For this review, take the finished solid that the model builds, in its own axes (mm). A direction names the side the tool comes from. Coordinates: 2 decimals unless noted, no trailing zeros. Order: outer loops, then holes, each group sorted by start corner. A loop starts at its lowest first (then second) coordinate and runs counter-clockwise, first axis right, second up. Notation, with made-up numbers: (73, -22.5) -> (103, -22.5) arc R5 cw to (103, -14.5) -> close; hole circle Ø11 at (75, 12). An arc over 180 degrees is marked (long way). Return JSON: item names as keys, results as strings. Group by question number.
Item 1: Take a section at B-B (y = 40). Write out the cut boundary in (x, z).
Item 2: Take a section at C-C (x = 40). Write out the cut boundary in (y, z), then the cut area to 3 significant figures.
Item 3: For line 1 along Y through (x, z) = (40, 5.5); line 2 along X through (y, z) = (40, 5.75); line 3 along Y through (x, z) = (72.5, 4.5), list the stretches that pass through material, from the lowest coordinate up.
Item 4: Machinability: for faces 4 (the flat face through (2, 33.5, 7)), 5 (the cylindrical face through (21.502, 64.787, 6.549)), 6 (the cylindrical face through (2, 79, 5)), which of the approach directions +Z, -Z, +X, -X, +Y, -Y give a long, thin tool a straight path to every point of the face, cutting with its end or side? Answer none if there is none.
Item 5: Take a section at A-A (z = 7.25). Write out the cut boundary in (x, y).
Item 6: Take a section at D-D (x = 73). Write out the cut boundary in (y, z).
Item 7: Draft analysis for pull direction Y (two halves, no side actions). For faces 1 (the flat face through (38, 41, 3)), 2 (the flat face through (40, 80, 5)), 3 (the flat face through (80, 40, 5)), state which applies: +Y half, -Y half, draft (parallel to the pull), parting line (faces both ways), or undercut.
Item 8: Insertion check: pin 1 (1.8 mm diameter, centred on x = 2, z = 6, fed in from -Y). The pin has a flat end and moves straight along its axis. Give the tip position at first contact, or say it passes through.
```python
from build123d import *

# Parameters (mm, degrees)
F1_DEPTH = 10
F3_DEPTH = 7
F4_R     = 37
F4_R_2   = 35.5
F5_DEPTH = 7
F6_W     = 20.75
F6_H     = 14
F7_DEPTH = 7


with BuildPart() as f1:
    # F0 (on Top) → F1 (new body)
    with BuildSketch(Plane.XY):
        with BuildLine():
            Line((75, 80), (5, 80))
            ThreePointArc((5, 80), (1.464466, 78.535534), (0, 75))
            Line((0, 75), (0, 5))
            ThreePointArc((0, 5), (1.464466, 1.464466), (5, 0))
            Line((5, 0), (75, 0))
            ThreePointArc((75, 0), (78.535534, 1.464466), (80, 5))
            Line((80, 5), (80, 75))
            ThreePointArc((80, 75), (78.535534, 78.535534), (75, 80))
        make_face()
    extrude(amount=F1_DEPTH)

    # F2 (on face) → F3 (cut)
    with BuildSketch(Plane.XY.offset(10)):
        with BuildLine():
            ThreePointArc((20.75, 17), (21.482233, 15.232233), (23.25, 14.5))
            Line((23.25, 14.5), (57.75, 14.5))
            ThreePointArc((57.75, 14.5), (59.517767, 15.232233), (60.25, 17))
            Line((60.25, 17), (60.25, 63))
            ThreePointArc((60.25, 63), (59.517767, 64.767767), (57.75, 65.5))
            Line((57.75, 65.5), (23.25, 65.5))
            ThreePointArc((23.25, 65.5), (21.482233, 64.767767), (20.75, 63))
            Line((20.75, 63), (20.75, 17))
        make_face()
    extrude(amount=-F3_DEPTH, mode=Mode.SUBTRACT)

    # F4 (on face) → F5 (cut)
    with BuildSketch(Plane.XY.offset(10)):
        with Locations((40, 40)):
            Circle(F4_R)
        with Locations((40, 40)):
            Circle(F4_R_2, mode=Mode.SUBTRACT)
    extrude(amount=-F5_DEPTH, mode=Mode.SUBTRACT)

    # F6 (on face) → F7 (cut)
    with BuildSketch(Plane.XY.offset(10)):
        with Locations((10.375, 26.5)):
            Rectangle(F6_W, F6_H)
    extrude(amount=-F7_DEPTH, mode=Mode.SUBTRACT)


solid = f1.part
```
Findings below:
{
 "1": {"outline": "(0, 0) -> (80, 0) -> (80, 10) -> (77, 10) -> (77, 3) -> (75.5, 3) -> (75.5, 10) -> (60.25, 10) -> (60.25, 3) -> (20.75, 3) -> (20.75, 10) -> (4.5, 10) -> (4.5, 3) -> (3, 3) -> (3, 10) -> (0, 10) -> close"},
 "2": {"outline": "(0, 0) -> (80, 0) -> (80, 10) -> (77, 10) -> (77, 3) -> (75.5, 3) -> (75.5, 10) -> (65.5, 10) -> (65.5, 3) -> (14.5, 3) -> (14.5, 10) -> (4.5, 10) -> (4.5, 3) -> (3, 3) -> (3, 10) -> (0, 10) -> close", "area": "422 mm2"},
 "3": {"line 1": "y = 0 to 3, 4.5 to 14.5, 65.5 to 75.5, 77 to 80", "line 2": "x = 0 to 3, 4.5 to 20.75, 60.25 to 75.5, 77 to 80", "line 3": "y = 0 to 22.32, 25.72 to 54.28, 57.68 to 80"},
 "4": {"face 4": "+Z, -X", "face 5": "+Z", "face 6": "+Z, -Z, -X, +Y"},
 "5": {"outline": "(0, 5) arc R5 ccw to (5, 0) -> (75, 0) arc R5 ccw to (80, 5) -> (80, 75) arc R5 ccw to (75, 80) -> (5, 80) arc R5 ccw to (0, 75) -> (0, 33.5) -> (3.58, 33.5) arc R37 cw (long way) to (9.2, 19.5) -> (0, 19.5) -> close; (5.1, 33.5) -> (20.75, 33.5) -> (20.75, 63) arc R2.5 cw to (23.25, 65.5) -> (57.75, 65.5) arc R2.5 cw to (60.25, 63) -> (60.25, 17) arc R2.5 cw to (57.75, 14.5) -> (23.25, 14.5) arc R2.5 cw to (20.75, 17) -> (20.75, 19.5) -> (11.02, 19.5) arc R35.5 ccw (long way) to start"},
 "6": {"outline": "(0, 0) -> (80, 0) -> (80, 10) -> (56.73, 10) -> (56.73, 3) -> (53.09, 3) -> (53.09, 10) -> (26.91, 10) -> (26.91, 3) -> (23.27, 3) -> (23.27, 10) -> (0, 10) -> close"},
 "7": {"face 1": "undercut", "face 2": "+Y half", "face 3": "draft"},
 "8": {"pin 1": "stops at y = 0.46"}
}
